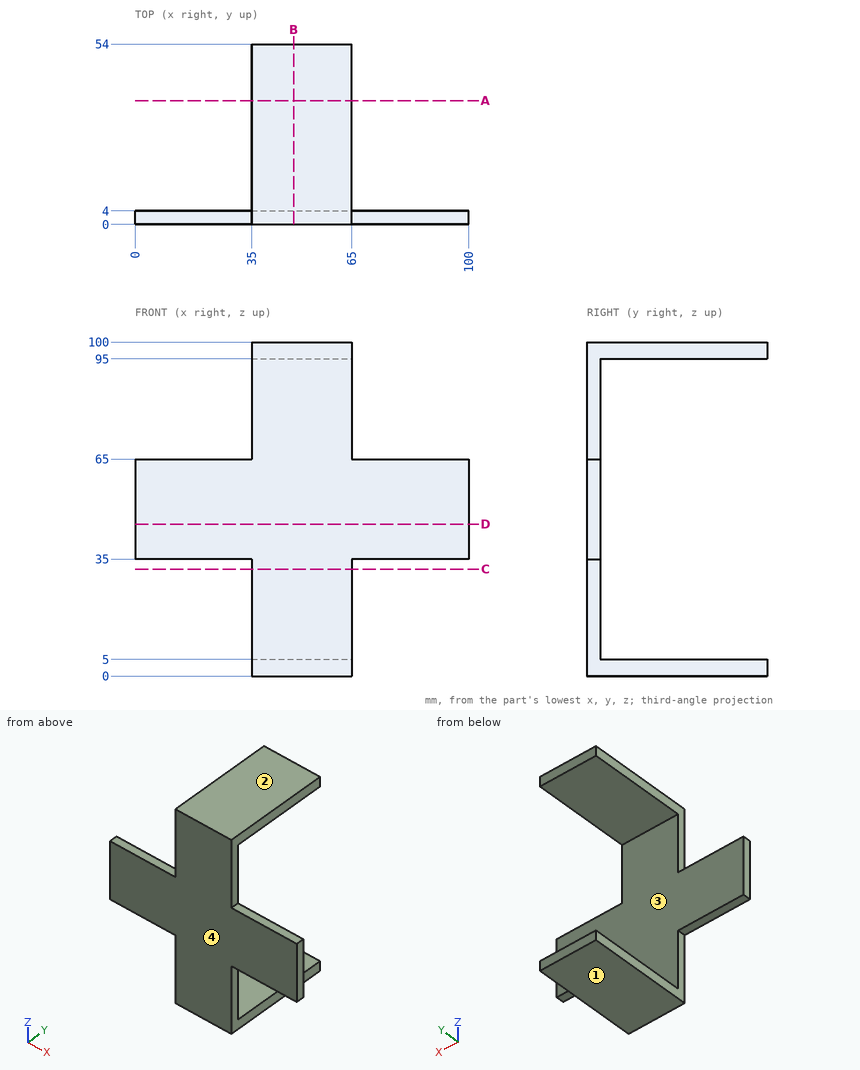
Here's the drawing with two shaded views (mm, measured from the low corner). I have some questions. Coordinates: 2 decimals unless noted, no trailing zeros. Order: outer loops, then holes, each group sorted by start corner. A loop starts at its lowest first (then second) coordinate and runs counter-clockwise, first axis right, second up.
Item 1: I need wall thicknesses on probe 1 along Z at (x, y) = (60.5, 13.5); probe 2 along Z at (x, y) = (26, 2.5); probe 3 along Y at (x, z) = (78, 43). Which ranges of each line are inside material? Lowest first, please.
Response values:
probe 1: z = 0 to 5, 95 to 100
probe 2: z = 35 to 65
probe 3: y = 0 to 4
Item 2: Thinking about a two-plate mould opening in Z: for the marked faces 1, 2, 3 and 4, which applies, pulls with the +Z half, pulls with the -Z half, needs draft (parallel to the pull), parting line crosses it, or undercut?
Response values:
face 1: pulls with the -Z half
face 2: pulls with the +Z half
face 3: undercut
face 4: needs draft
Item 3: If we section it at D-D, the plane z = 45.5: List the corners of the cut face in (x, y) for me.
Response values:
outline: (0, 0) - (100, 0) - (100, 4) - (0, 4) - close
Item 4: I'm going to push flat-ended pins straight in: pin 1 Ø4.5 at (x, y) = (83, 2.5) entering from -Z; pin 2 Ø1.2 at (x, y) = (10, 2.5) entering from +Z. Where does each tip first touch, or does it pass through?
Response values:
pin 1: stops at z = 35
pin 2: stops at z = 65
Item 5: If we section it at B-B, the plane x = 47.5: List the corners of the cut face in (y, z) for me.
Response values:
outline: (0, 0) - (54, 0) - (54, 5) - (4, 5) - (4, 95) - (54, 95) - (54, 100) - (0, 100) - close
Item 6: If we section it at C-C, the plane z = 32: List the corners of the cut face in (x, y) for me.
Response values:
outline: (35, 0) - (65, 0) - (65, 4) - (35, 4) - close
Item 7: If we section it at A-A, the plane y = 37: List the corners of the cut face in (x, z) for me, then the cut area to 3 significant figures.
Response values:
outline: (35, 0) - (65, 0) - (65, 5) - (35, 5) - close; (35, 95) - (65, 95) - (65, 100) - (35, 100) - close
area: 300 mm2
